from build123d import *

# Parameters (mm, degrees)
CROQUIS1_W              = 46.6
CROQUIS1_H              = 11.5
CROQUIS1_W_2            = 8
CROQUIS1_H_2            = 72
SALIENTE_EXTRUIR1_DEPTH = 25
CROQUIS3_W              = 30
CROQUIS3_H              = 5
CORTAR_EXTRUIR1_DEPTH   = 100
CROQUIS4_W              = 5
CROQUIS4_H              = 10
CORTAR_EXTRUIR2_DEPTH   = 2000
CORTAR_EXTRUIR3_DEPTH   = 2000
CROQUIS7_W              = 38.34522513
CROQUIS7_H              = 2.150988128
SALIENTE_EXTRUIR2_DEPTH = 90
CROQUIS8_W              = 13.2
CROQUIS8_H              = 10
CORTAR_EXTRUIR4_DEPTH   = 10
SALIENTE_EXTRUIR3_DEPTH = 95
CROQUIS10_R             = 12.5
CORTAR_EXTRUIR5_DEPTH   = 95
SALIENTE_EXTRUIR4_DEPTH = 2
REDONDEO1_R             = 10
CROQUIS13_R             = 1.5
CORTAR_EXTRUIR7_DEPTH   = 5
CROQUIS16_W             = 11.760768102
CROQUIS16_H             = 18.8
CORTAR_EXTRUIR9_DEPTH   = 10
CORTAR_EXTRUIR10_DEPTH  = 10
CROQUIS18_W             = 27
CROQUIS18_H             = 4
CORTAR_EXTRUIR11_DEPTH  = 10
CROQUIS20_R             = 1.5
CORTAR_EXTRUIR12_DEPTH  = 10


with BuildPart() as part:
    # Croquis1 → Saliente-Extruir1 (new body)
    with BuildSketch(Plane.XY):
        with Locations((9.10717527, 8.346927266)):
            Rectangle(CROQUIS1_W, CROQUIS1_H)
        with Locations((28.40717527, -33.403072734)):
            Rectangle(CROQUIS1_W_2, CROQUIS1_H_2)
        Polygon((32.40717527, -80.903072734), (32.40717527, -69.403072734), (24.40717527, -69.403072734), (-14.19282473, -69.403072734), (-14.19282473, -80.903072734), align=None)
    extrude(amount=SALIENTE_EXTRUIR1_DEPTH)

    # Croquis3 → Cortar-Extruir1 (cut)
    with BuildSketch(Plane(origin=(32.40717527, 0, 0), x_dir=(0, 0, -1), z_dir=(1, 0, 0))):
        with Locations((-30, -60.403072734)):
            Rectangle(CROQUIS3_W, CROQUIS3_H)
        with Locations((-30, -6.403072734)):
            Rectangle(CROQUIS3_W, CROQUIS3_H)
    extrude(amount=-CORTAR_EXTRUIR1_DEPTH, mode=Mode.SUBTRACT)

    # Croquis4 → Cortar-Extruir2 (cut)
    with BuildSketch(Plane(origin=(0, -80.903072734, 0), x_dir=(-1, 0, 0), z_dir=(0, -1, 0))):
        with Locations((-5.979621663, -20)):
            Rectangle(CROQUIS4_W, CROQUIS4_H)
    extrude(amount=-CORTAR_EXTRUIR2_DEPTH, mode=Mode.SUBTRACT)

    # Croquis5 → Cortar-Extruir3 (cut)
    with BuildSketch(Plane.XZ.offset(80.903072734)):
        Polygon((32.40717527, 0), (26.484562574, 25), (32.40717527, 25), align=None)
    extrude(amount=-CORTAR_EXTRUIR3_DEPTH, mode=Mode.SUBTRACT)

    # Croquis7 → Saliente-Extruir2 (add)
    with BuildSketch(Plane(origin=(0, 14.096927266, 0), x_dir=(1, 0, 0), z_dir=(0, 1, 0))):
        with Locations((4.979787835, -1.075494064)):
            Rectangle(CROQUIS7_W, CROQUIS7_H)
    extrude(amount=-SALIENTE_EXTRUIR2_DEPTH)

    # Croquis8 → Cortar-Extruir4 (cut)
    with BuildSketch(Plane(origin=(0, 0, 0), x_dir=(-1, 0, 0), z_dir=(0, 0, -1))):
        with Locations((-21.60717527, 2.096927266)):
            Rectangle(CROQUIS8_W, CROQUIS8_H)
        with Locations((-21.60717527, -68.903072734)):
            Rectangle(CROQUIS8_W, CROQUIS8_H)
    extrude(amount=-CORTAR_EXTRUIR4_DEPTH, mode=Mode.SUBTRACT)

    # Croquis9 → Saliente-Extruir3 (add)
    with BuildSketch(Plane.XZ.offset(80.903072734)):
        Polygon((32.40717527, 0), (34.40717527, 0), (29.871577543, 10.70303706), align=None)
    extrude(amount=-SALIENTE_EXTRUIR3_DEPTH)

    # Croquis10 → Cortar-Extruir5 (cut)
    with BuildSketch(Plane.XZ.offset(80.903072734)):
        with Locations((-23.100515524, 11.30775419)):
            Circle(CROQUIS10_R)
    extrude(amount=-CORTAR_EXTRUIR5_DEPTH, mode=Mode.SUBTRACT)

    # Croquis11 → Saliente-Extruir4 (add)
    with BuildSketch(Plane(origin=(30.685017166, 0, 7.26941889), x_dir=(0.2305238801243756, 0, -0.9730666681643158), z_dir=(0.9730666681643156, 0, 0.23052388012437558))):
        with BuildLine():
            Line((-11.378913607, -34.525526143), (-17.390636934, -47.778099529))
            ThreePointArc((-17.390636934, -47.778099529), (-5.898546533, -45.001394179), (-11.378913607, -34.525526143))
        make_face()
        with BuildLine():
            Line((-11.378913607, -32.280619326), (-17.390636934, -19.028045939))
            ThreePointArc((-17.390636934, -19.028045939), (-5.898546533, -21.804751289), (-11.378913607, -32.280619326))
        make_face()
    extrude(amount=SALIENTE_EXTRUIR4_DEPTH)

    # Redondeo1
    redondeo1_edges = [part.edges().sort_by_distance(p)[0] for p in [
        (29.871577543, -33.403072734, 10.70303706),
    ]]
    fillet(redondeo1_edges, radius=REDONDEO1_R)

    # Croquis13 → Cortar-Extruir7 (cut)
    with BuildSketch(Plane(origin=(0, 0, 0), x_dir=(-1, 0, 0), z_dir=(0, 0, -1))):
        with Locations((-18.80717527, -77.903072734)):
            Circle(CROQUIS13_R)
        with Locations((1.89282473, -77.903072734)):
            Circle(CROQUIS13_R)
        with Locations((-29.560114376, -45.103072734)):
            Circle(CROQUIS13_R)
        with Locations((-29.560114376, -21.703072734)):
            Circle(CROQUIS13_R)
        with Locations((-18.80717527, 11.096927266)):
            Circle(CROQUIS13_R)
        with Locations((1.89282473, 11.096927266)):
            Circle(CROQUIS13_R)
    extrude(amount=-CORTAR_EXTRUIR7_DEPTH, mode=Mode.SUBTRACT)

    # Croquis16 → Cortar-Extruir9 (cut)
    with BuildSketch(Plane(origin=(30.685017166, 0, 7.26941889), x_dir=(0.2305238801243756, 0, -0.9730666681643158), z_dir=(0.9730666681643156, 0, 0.23052388012437558))):
        with Locations((-13.601726627, -60.013945982)):
            Rectangle(CROQUIS16_W, CROQUIS16_H)
        with Locations((-13.601726627, -6.792199486)):
            Rectangle(CROQUIS16_W, CROQUIS16_H)
    extrude(amount=-CORTAR_EXTRUIR9_DEPTH, mode=Mode.SUBTRACT)

    # Croquis17 → Cortar-Extruir10 (cut)
    with BuildSketch(Plane.XY.offset(25)):
        Polygon((24.40717527, -69.403072734), (24.40717527, -74.103072734), (22.50717527, -74.103072734), (22.50717527, -69.413945982), align=None)
        Polygon((22.50717527, 2.607800514), (24.40717527, 2.596927266), (24.40717527, 7.296927266), (22.50717527, 7.296927266), align=None)
    extrude(amount=-CORTAR_EXTRUIR10_DEPTH, mode=Mode.SUBTRACT)

    # Croquis18 → Cortar-Extruir11 (cut)
    with BuildSketch(Plane.XY.offset(25)):
        Polygon((3.479621663, -80.903072734), (3.479621663, -79.103072734), (-0.341573642, -80.903072734), align=None)
        Polygon((8.479621663, -80.903072734), (8.457050966, -79.103072734), (12.278246271, -80.903072734), align=None)
        with Locations((5.979621663, 10.296927266)):
            Rectangle(CROQUIS18_W, CROQUIS18_H)
        Polygon((12.278246271, 14.096927266), (8.479621663, 14.096927266), (8.457050966, 12.296927266), align=None)
        with Locations((5.979621663, -77.103072734)):
            Rectangle(CROQUIS18_W, CROQUIS18_H)
        Polygon((3.479621663, 12.296927266), (-0.341573642, 14.096927266), (3.479621663, 14.096927266), align=None)
    extrude(amount=-CORTAR_EXTRUIR11_DEPTH, mode=Mode.SUBTRACT)

    # Croquis20 → Cortar-Extruir12 (cut)
    with BuildSketch(Plane.XY.offset(25)):
        with Locations((11.463707662, -73.403072734)):
            Circle(CROQUIS20_R)
        with Locations((-6.881069151, -73.403072734)):
            Circle(CROQUIS20_R)
        with Locations(Location((11.463707662, 6.596927266, 0), (0, 0, 180))):
            Circle(CROQUIS20_R)
        with Locations(Location((-6.881069151, 6.596927266, 0), (0, 0, 180))):
            Circle(CROQUIS20_R)
    extrude(amount=-CORTAR_EXTRUIR12_DEPTH, mode=Mode.SUBTRACT)


solid = part.part
Verification items for the finished model (mm, model axes). A direction names the side the tool comes from. Coordinates: 2 decimals unless noted, no trailing zeros. Write each loop counter-clockwise with the first axis right and the second up, starting at its lowest first coordinate (ties: lowest second). Pieces come first, ordered by that corner, then holes. Notation, with made-up numbers: (42, 80) - (100, 80) arc R28 ccw to (100, 107) - close; hole circle Ø9 at (85.25, 12). An arc over 180 degrees is marked (long way). Answer as a JSON object with one key per item and string values.
(1) Tool access check on faces 4 (the flat face through (14, 12.297, 20)), 5 (the flat face through (8.48, -72, 20)), 6 (the flat face through (15.007, 4, 4)), 7 (the flat face through (5, -33, 2.151)). Record the directions out of +Z, -Z, +X, -X, +Y, -Y that give a thin tool (end or side, any length) a straight path to the whole face; none if there is none.
Report:
{"face 4": "+Z", "face 5": "+Z, +Y, -Y", "face 6": "-Z", "face 7": "+Z, -X"}
(2) Cross-section at D-D on y = -25.5. Record the cut outline in (x, z).
Report:
{"outline": "(-14.19, 0) - (24.15, 0) - (24.15, 2.15) - (-14.19, 2.15) - close; (24.41, 0) - (34.41, 0) - (30.2, 9.93) arc R10 cw to (29.68, 11.52) - (29.47, 12.38) - (31.42, 12.84) - (29.3, 21.8) - (27.35, 21.33) - (26.48, 25) - (24.41, 25) - close"}
(3) Mould release check, pull along Z, two halves, no side actions. Record for faces 1 (the flat face through (11, 7, 15)), 2 (the flat face through (20, -2.903, 1)), 3 (the cylindrical face through (30.266, -45.174, 13.315)): pulls with the +Z half, pulls with the -Z half, needs draft (parallel to the pull), parting line crosses it, or undercut.
Report:
{"face 1": "pulls with the +Z half", "face 2": "needs draft", "face 3": "undercut"}
(4) Gauge pin test, flat ends, axial feed: pin 1 Ø2.5 at (x, y) = (11.5, -73.5) entering from +Z; pin 2 Ø8 at (y, z) = (-7.5, 17) entering from +X; pin 3 Ø3 at (y, z) = (-77, 19) entering from +X. Record the tip position at first contact, or that the pin passes through.
Report:
{"pin 1": "z = 15", "pin 2": "x = 29.33", "pin 3": "x = 28.26"}
(5) Cross-section at C-C on z = 7.75. Record the cut outline in (x, y).
Report:
{"outline": "(-11.12, -80.9) - (31.12, -80.9) - (31.12, 14.1) - (-11.12, 14.1) - (-11.12, 2.6) - (15.01, 2.6) - (15.01, 7.1) - (28.21, 7.1) - (28.21, -2.9) - (24.41, -2.9) - (24.41, -63.9) - (28.21, -63.9) - (28.21, -73.9) - (15.01, -73.9) - (15.01, -69.4) - (-11.12, -69.4) - close"}
(6) Cross-section at B-B on x = 6. Record the cut outline in (y, z), plus the area to 3 significant figures.
Report:
{"outline": "(-80.9, 0) - (14.1, 0) - (14.1, 15) - (2.6, 15) - (2.6, 2.15) - (-69.4, 2.15) - (-69.4, 15) - (-80.9, 15) - close", "area": "500 mm^2"}
(7) Thickness scan on line 1 along Y through (x, z) = (-4, 22.75); line 2 along Y through (x, z) = (1, 7.75); line 3 along X through (y, z) = (5.5, 16.75). Record the ranges inside material, lowest first.
Report:
{"line 1": "-80.9 to -79.1, -75.1 to -69.4, 2.6 to 8.3, 12.3 to 14.1", "line 2": "-80.9 to -69.4, 2.6 to 14.1", "line 3": "-11.85 to -7.9, -5.86 to 3.48, 8.48 to 10.44, 12.49 to 22.51, 24.41 to 28.44"}
(8) Cross-section at A-A on y = -58.5. Record the cut outline in (x, z), plus the area to 3 significant figures.
Report:
{"outline": "(-14.19, 0) - (24.15, 0) - (24.15, 2.15) - (-14.19, 2.15) - close; (24.41, 0) - (34.41, 0) - (30.2, 9.93) arc R10 cw to (29.68, 11.52) - (28.91, 14.78) - (24.41, 13.72) - close", "area": "183 mm^2"}
